from build123d import *

# Parameters (mm, degrees)
SKETCH1_R           = 23.495
SKETCH1_R_2         = 12.065
BOSS_EXTRUDE1_DEPTH = 38.1
CUT_EXTRUDE1_START  = -31.75
SKETCH2_R           = 15.24
SKETCH2_R_2         = 12.065
CUT_EXTRUDE1_DEPTH  = 31.75
SKETCH4_R           = 2.54
CUT_EXTRUDE5_DEPTH  = 5.08


with BuildPart() as part:
    # Sketch1 → Boss-Extrude1 (new body)
    with BuildSketch(Plane.XY):
        Circle(SKETCH1_R)
        Circle(SKETCH1_R_2, mode=Mode.SUBTRACT)
    extrude(amount=-BOSS_EXTRUDE1_DEPTH)

    # Sketch2 → Cut-Extrude1 (cut)
    with BuildSketch(Plane(origin=(0, 0, -38.1), x_dir=(-1, 0, 0), z_dir=(0, 0, -1)).offset(CUT_EXTRUDE1_START)):
        Circle(SKETCH2_R)
        with Locations(Location((0, 0, 0), (0, 0, 180))):
            Circle(SKETCH2_R_2, mode=Mode.SUBTRACT)
    extrude(amount=CUT_EXTRUDE1_DEPTH, mode=Mode.SUBTRACT)

    # Sketch4 → Cut-Extrude5 (cut)
    with BuildSketch(Plane(origin=(0, 0, -38.1), x_dir=(-1, 0, 0), z_dir=(0, 0, -1))):
        with Locations((0, 19.3675)):
            Circle(SKETCH4_R)
        with Locations((0, -19.3675)):
            Circle(SKETCH4_R)
    extrude(amount=-CUT_EXTRUDE5_DEPTH, mode=Mode.SUBTRACT)


solid = part.part
For this review, take the finished solid that the model builds, in its own axes (mm). A direction names the side the tool comes from. Round coordinates to 2 decimals unless told otherwise and drop trailing zeros. Loops run counter-clockwise (first coordinate to the right, second up) from the corner with the lowest first, then second, coordinate; pieces in that order, holes last. Notation, with made-up numbers: (-20.75, 78) - (25.25, 78) arc R13 ccw to (25.25, 88) - close; hole circle Ø11 at (4.5, 8.25). An arc over 180 degrees is marked (long way). One line per question, with ' | ' between items.
Q1. Take a section at D-D (y = 14.5). Give the boundary of the cut face in (x, z), and give its area (3 significant figures).
Taken from the geometry:
outline: (-18.49, -38.1) - (-4.69, -38.1) - (-4.69, -6.35) - (4.69, -6.35) - (4.69, -38.1) - (18.49, -38.1) - (18.49, 0) - (-18.49, 0) - close | area: 1,110 mm²
Q2. For pin 1 (12 mm diameter, centred on y = -13.5, z = -19.5, fed in from +X); pin 2 (4 mm diameter, centred on x = 0, y = 19.37, fed in from -Z); pin 3 (4 mm diameter, centred on x = 16, z = -15.5, fed in from -Y); pin 4 (9 mm diameter, centred on x = 5.5, y = 2, fed in from -Z), all flat-tipped, find the tip position at first contact; note any pin that passes through.
Taken from the geometry:
pin 1: stops at x = 22.27 | pin 2: stops at z = -33.02 | pin 3: stops at y = -18.87 | pin 4: passes through
Q3. The part is to be moulded in two halves that separate along Y. For faces 1 (the flat face through (-11, 6, 0)), 2 (the flat face through (0, 19, -33.02)), 3 (the cylindrical face through (-5.093, -22.936, -18.783)), say which applies: released by +Y, released by -Y, zero draft, split by the parting line, or undercut.
Taken from the geometry:
face 1: zero draft | face 2: undercut | face 3: split by the parting line
Q4. Take a section at C-C (z = -5). Give the boundary of the cut face in (x, y) (3 decimals), and give its area (3 significant figures).
Taken from the geometry:
outline: circle Ø46.99 at (0, 0); hole circle Ø24.13 at (0, 0) | area: 1,280 mm²
Q5. Tool access review of faces 4 (the flat face through (5, -15, -38.1)), 5 (the cylindrical face through (0.331, 21.886, -35.596)): name each direction out of +Z, -Z, +X, -X, +Y, -Y from which nothing blocks a thin tool from reaching the whole face with its end or side.
Taken from the geometry:
face 4: -Z, +X, -X, +Y, -Y | face 5: -Z
Q6. Take a section at A-A (y = 0). Give the boundary of the cut face in (x, z) (3 decimals), and give its area (3 significant figures).
Taken from the geometry:
outline: (-23.495, -38.1) - (-15.24, -38.1) - (-15.24, -6.35) - (-12.065, -6.35) - (-12.065, 0) - (-23.495, 0) - close; (12.065, -6.35) - (15.24, -6.35) - (15.24, -38.1) - (23.495, -38.1) - (23.495, 0) - (12.065, 0) - close | area: 669 mm²
Q7. For line 1 along Y through (x, z) = (0, -36.9) (1 decimal); line 2 along Y through (x, z) = (6.5, -32); line 3 along X through (y, z) = (-8, -23), list the stretches that pass through material, from the lowest coordinate up. Write a range as [from, to].
Taken from the geometry:
line 1: y = [-23.5, -21.9], [-16.8, -15.2], [15.2, 16.8], [21.9, 23.5] | line 2: y = [-22.58, -13.78], [13.78, 22.58] | line 3: x = [-22.09, -12.97], [12.97, 22.09]
